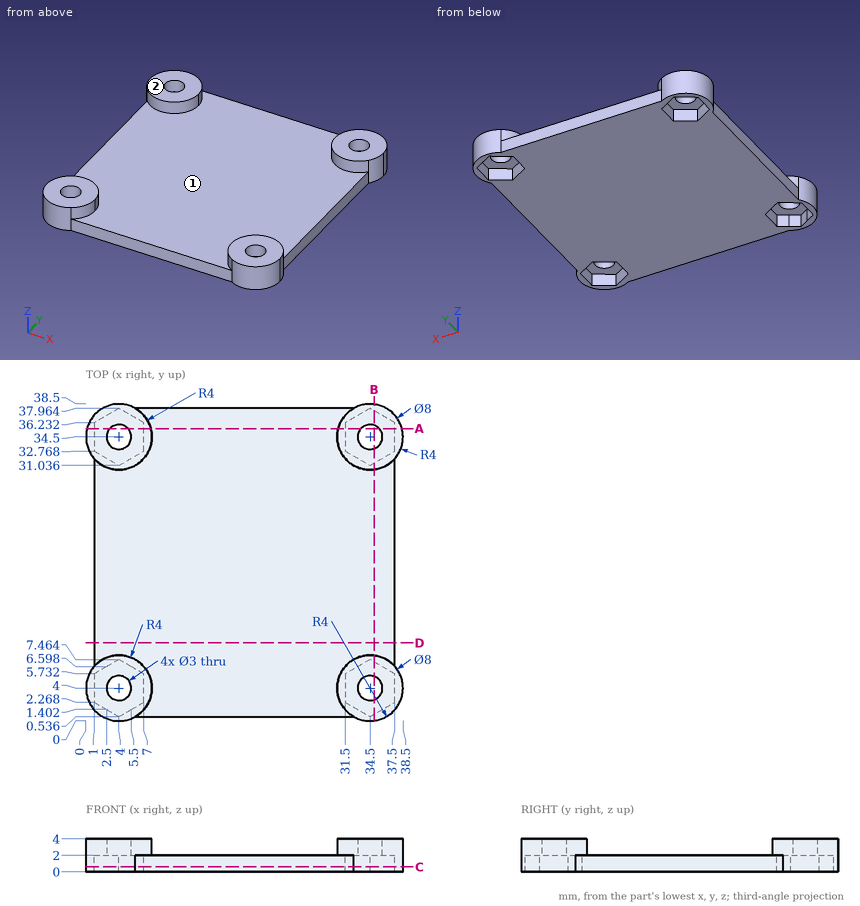
Can you work these out from the drawing? Everything is in mm from the part's minimum corner. A direction names the side the tool comes from. Round coordinates to 2 decimals unless told otherwise and drop trailing zeros. Write each loop counter-clockwise with the first axis right and the second up, starting at its lowest first coordinate (ties: lowest second). Pieces come first, ordered by that corner, then holes. Notation, with made-up numbers: M -36.75,16 L 5.25,16 A24 cw 5.25,46 Z; hole C 46.5,-32 d7. An arc over 180 degrees is marked long. Use a Markdown table: item, result.
Item 1: If I drill on line 1 along Y through (x, z) = (4, 2.7); line 2 along X through (y, z) = (34.5, 0.35), over which ranges is the centre line in solid material (lowest first)? Write a range as [from, to].
Found:
| item | result |
|---|---|
| line 1 | y = [0, 2.5], [5.5, 8], [30.5, 33], [36, 38.5] |
| line 2 | x = [0, 1], [7, 31.5], [37.5, 38.5] |
Item 2: I want a section at B-B (x = 35). List the corners of the cut face in (y, z) for me, and give its area (3 significant figures).
Found:
| item | result |
|---|---|
| outline | M 0.03,0 L 0.82,0 L 0.82,2 L 2.59,2 L 2.59,4 L 0.03,4 Z; M 5.41,2 L 7.18,2 L 7.18,0 L 31.32,0 L 31.32,2 L 33.09,2 L 33.09,4 L 30.53,4 L 30.53,2 L 7.97,2 L 7.97,4 L 5.41,4 Z; M 35.91,2 L 37.68,2 L 37.68,0 L 38.47,0 L 38.47,4 L 35.91,4 Z |
| area | 71.9 mm2 |
Item 3: I want a section at A-A (y = 35.5). List the corners of the cut face in (x, z) for me.
Found:
| item | result |
|---|---|
| outline | M 0.13,0 L 1,0 L 1,2 L 2.88,2 L 2.88,4 L 0.13,4 Z; M 5.12,2 L 7,2 L 7,0 L 31.5,0 L 31.5,2 L 33.38,2 L 33.38,4 L 30.63,4 L 30.63,2 L 7.87,2 L 7.87,4 L 5.12,4 Z; M 35.62,2 L 37.5,2 L 37.5,0 L 38.37,0 L 38.37,4 L 35.62,4 Z |
Item 4: I want a section at C-C (z = 0.6). State how many separate pieces and enclosed holes the cut face has, and give its area (3 significant figures).
Found:
| item | result |
|---|---|
| separate pieces | 1 |
| enclosed holes | 4 |
| area | 1,260 mm2 |
Item 5: I want a section at D-D (y = 9.5). List the corners of the cut face in (x, z) for me.
Found:
| item | result |
|---|---|
| outline | M 1,0 L 37.5,0 L 37.5,2 L 1,2 Z |
Item 6: For pin 1 Ø5 at (x, y) = (4, 4) entering from -Z; pin 2 Ø1.6 at (x, z) = (20.5, 1) entering from +Y; pin 3 Ø0.6 at (y, z) = (3.5, 1) entering from -X (3 decimals), each with a flat end and sliding along its axis, tell me the tip position at first contact or that it passes through.
Found:
| item | result |
|---|---|
| pin 1 | stops at z = 2 |
| pin 2 | stops at y = 37.96 |
| pin 3 | stops at x = 0.005 |
Item 7: Which directions (+Z, -Z, +X, -X, +Y, -Y) give clear straight access to the entire face, cutting with the end or side of a thin tool? Please do the marked faces 1 and 2.
Found:
| item | result |
|---|---|
| face 1 | +Z |
| face 2 | +Z, +X, -X, +Y, -Y |
